```python
from build123d import *

# Parameters (mm, degrees)
F1_DEPTH  = 25
F3_DEPTH  = 3
F4_R      = 2
F5_R      = 4
F6_W      = 25
F6_H      = 25
F7_DEPTH  = 25
F8_R      = 3
F9_R      = 4.5
F10_DEPTH = 25


with BuildPart() as f1:
    # F0 (on Front) → F1 (new body)
    with BuildSketch(Plane.XZ):
        Polygon((13.834733, 33.4), (-13.834733, 33.4), (-33.4, 13.834733), (-33.4, -13.834733), (-13.834733, -33.4), (13.834733, -33.4), (33.4, -13.834733), (33.4, 13.834733), align=None)
        Polygon((-12.592092, -30.4), (-30.4, -12.592092), (-30.4, 12.592092), (-12.592092, 30.4), (12.592092, 30.4), (30.4, 12.592092), (30.4, -12.592092), (12.592092, -30.4), align=None, mode=Mode.SUBTRACT)
    extrude(amount=F1_DEPTH)

    # F2 (on face) → F3 (join)
    with BuildSketch(Plane.XZ.offset(25)):
        Polygon((14.497475, 35), (-14.497475, 35), (-35, 14.497475), (-35, -14.497475), (-14.497475, -35), (14.497475, -35), (35, -14.497475), (35, 14.497475), align=None)
    extrude(amount=F3_DEPTH)

    # F4
    f4_edges = [f1.edges().sort_by_distance(p)[0] for p in [
        (13.834733, -12.5, 33.4),
        (33.4, -12.5, 13.834733),
        (33.4, -12.5, -13.834733),
        (13.834733, -12.5, -33.4),
        (-13.834733, -12.5, -33.4),
        (-33.4, -12.5, -13.834733),
        (-33.4, -12.5, 13.834733),
        (-13.834733, -12.5, 33.4),
        (-30.4, -12.5, 12.592092),
        (-30.4, -12.5, -12.592092),
        (-12.592092, -12.5, 30.4),
        (12.592092, -12.5, 30.4),
        (30.4, -12.5, 12.592092),
        (30.4, -12.5, -12.592092),
        (-12.592092, -12.5, -30.4),
        (12.592092, -12.5, -30.4),
    ]]
    fillet(f4_edges, radius=F4_R)

    # F5
    f5_edges = [f1.edges().sort_by_distance(p)[0] for p in [
        (-14.497475, -26.5, 35),
        (-35, -26.5, 14.497475),
        (14.497475, -26.5, 35),
        (35, -26.5, 14.497475),
        (35, -26.5, -14.497475),
        (14.497475, -26.5, -35),
        (-14.497475, -26.5, -35),
        (-35, -26.5, -14.497475),
    ]]
    fillet(f5_edges, radius=F5_R)

    # F6 (on face) → F7 (cut)
    with BuildSketch(Plane.XZ.offset(28)):
        Rectangle(F6_W, F6_H)
    extrude(amount=-F7_DEPTH, mode=Mode.SUBTRACT)

    # F8
    f8_edges = [f1.edges().sort_by_distance(p)[0] for p in [
        (-12.5, -26.5, 12.5),
        (12.5, -26.5, 12.5),
        (12.5, -26.5, -12.5),
        (-12.5, -26.5, -12.5),
    ]]
    fillet(f8_edges, radius=F8_R)

    # F9 (on face) → F10 (cut)
    with BuildSketch(Plane.XZ.offset(28)):
        with Locations((0, 22.5)):
            Circle(F9_R)
        with Locations((22.5, 0)):
            Circle(F9_R)
        with Locations((0, -22.5)):
            Circle(F9_R)
        with Locations((-22.5, 0)):
            Circle(F9_R)
    extrude(amount=-F10_DEPTH, mode=Mode.SUBTRACT)


solid = f1.part
```
The model under review builds one solid part; all positions refer to its coordinate system, in mm. A direction names the side the tool comes from. Give positions to 0.01 mm unless a question says otherwise; leave off trailing zeros. Loops run counter-clockwise (first coordinate to the right, second up) from the corner with the lowest first, then second, coordinate; pieces in that order, holes last. Notation, with made-up numbers: (82, 14.5) -> (104, 14.5) arc R10 cw to (104, 20.5) -> close; hole circle Ø7 at (-39.5, -26). An arc over 180 degrees is marked (long way). Use CSV: the item, a comma, the result in double quotes.
1. Consider section C-C, the plane x = 0. Write out the cut boundary in (y, z), then the cut area to 3 significant figures.
Result:
outline,"(-28, -35) -> (-25, -35) -> (-25, -33.4) -> (0, -33.4) -> (0, -30.4) -> (-25, -30.4) -> (-25, -27) -> (-28, -27) -> close; (-28, -18) -> (-25, -18) -> (-25, -12.5) -> (-28, -12.5) -> close; (-28, 12.5) -> (-25, 12.5) -> (-25, 18) -> (-28, 18) -> close; (-28, 27) -> (-25, 27) -> (-25, 30.4) -> (0, 30.4) -> (0, 33.4) -> (-25, 33.4) -> (-25, 35) -> (-28, 35) -> close"
area,"231 mm²"
2. For P1, Ø12.5, axis at x = 1, y = -15.5, coming from the -Z side; P2, Ø7, axis at x = 22.5, z = 0, coming from the -Y side; P3, Ø1, axis at x = 6.5, y = -9, coming from the +Z side; P4, Ø12, axis at y = -9, z = -27.5, coming from the -X side, all flat-tipped, find the tip position at first contact; note any pin that passes through.
Result:
P1,"stops at z = -33.4"
P2,"passes through"
P3,"stops at z = 33.4"
P4,"stops at x = -25.73"
3. Machinability: for faces 4 (the face through (11.64, -26.48, 11.6)), 5 (the face through (-34.687, -26.521, 14.392)), 6 (the face through (23.489, -12.325, -23.746)), 7 (the face through (34.687, -26.521, 14.392)), 8 (the face through (0, -12, 30.4)), which of the approach directions +Z, -Z, +X, -X, +Y, -Y give a long, thin tool a straight path to every point of the face, cutting with its end or side? Answer none if there is none.
Result:
face 4,"+Y, -Y"
face 5,"+Z, -X, +Y, -Y"
face 6,"-Z, +X, +Y"
face 7,"+Z, +X, +Y, -Y"
face 8,"+Y"
4. Consider section B-B, the plane z = 0. Write out the cut boundary in (x, y), then the cut area to 3 significant figures.
Result:
outline,"(-35, -28) -> (-27, -28) -> (-27, -25) -> (-30.4, -25) -> (-30.4, 0) -> (-33.4, 0) -> (-33.4, -25) -> (-35, -25) -> close; (-18, -28) -> (-12.5, -28) -> (-12.5, -25) -> (-18, -25) -> close; (12.5, -28) -> (18, -28) -> (18, -25) -> (12.5, -25) -> close; (27, -28) -> (35, -28) -> (35, -25) -> (33.4, -25) -> (33.4, 0) -> (30.4, 0) -> (30.4, -25) -> (27, -25) -> close"
area,"231 mm²"
5. Consider section D-D, the plane x = 8. Write out the cut boundary in (y, z), then the cut area to 3 significant figures.
Result:
outline,"(-28, -35) -> (-25, -35) -> (-25, -33.4) -> (0, -33.4) -> (0, -30.4) -> (-25, -30.4) -> (-25, -12.5) -> (-28, -12.5) -> close; (-28, 12.5) -> (-25, 12.5) -> (-25, 30.4) -> (0, 30.4) -> (0, 33.4) -> (-25, 33.4) -> (-25, 35) -> (-28, 35) -> close"
area,"285 mm²"
6. To check wall thickness, follow probe 1 along Z at (x, y) = (0, -26.3); probe 2 along Z at (x, y) = (-4, -23.75). State the ranges of each line that lie inside material, in increasing order. Write a range as from..to.
Result:
probe 1,"z = -35..-27, -18..-12.5, 12.5..18, 27..35"
probe 2,"z = -33.4..-30.4, 30.4..33.4"
7. The part is to be moulded in two halves that separate along X. For faces 1 (the face through (-23.489, -12.325, 23.746)), 2 (the face through (14.392, -26.521, -34.687)), 3 (the face through (-30.4, -12, 0)), say which applies: +X half, -X half, draft (parallel to the pull), parting line (faces both ways), or undercut.
Result:
face 1,"-X half"
face 2,"+X half"
face 3,"undercut"
